CAD build for the part. Positions are in the model's coordinates, mm. Round coordinates to 2 decimals unless told otherwise and drop trailing zeros. Write each loop counter-clockwise with the first axis right and the second up, starting at its lowest first coordinate (ties: lowest second). Pieces come first, ordered by that corner, then holes. Notation, with made-up numbers: (-3, -39) - (25, -39) arc R27 ccw to (25, -2) - close; hole circle Ø7 at (-10, -40). An arc over 180 degrees is marked (long way). Use one line per item in the form item = value. Start each with the question number.
Item 1: Pin check, flat tips, straight feed: pin 1 (5.5 mm diameter, centred on x = -22, z = 217.92, fed in from -Y); pin 2 (2 mm diameter, centred on y = 83, z = 282, fed in from +X); pin 3 (2 mm diameter, centred on x = -8.5, z = 222.5, fed in from -Y). Stop position of each tip, or through.
Item 2: Band-saw the part on B-B, the plane z = 260. List the corners of the cut face in (x, y), and give its area (3 significant figures).
Item 3: Drill centre lines: L1, parallel to X at y = 80.9, z = 303; L2, parallel to Z at x = -35, y = 81.4; L3, parallel to Z at x = 16, y = 80.25. Where is each one in solid material? Low to high.
Item 4: Band-saw the part on D-D, the plane x = 2.5. List the corners of the cut face in (y, z).
Item 5: Band-saw the part on A-A, the plane x = 22. Give the number of separate pieces and of enclosed holes in the cut face, and give its area (3 significant figures).
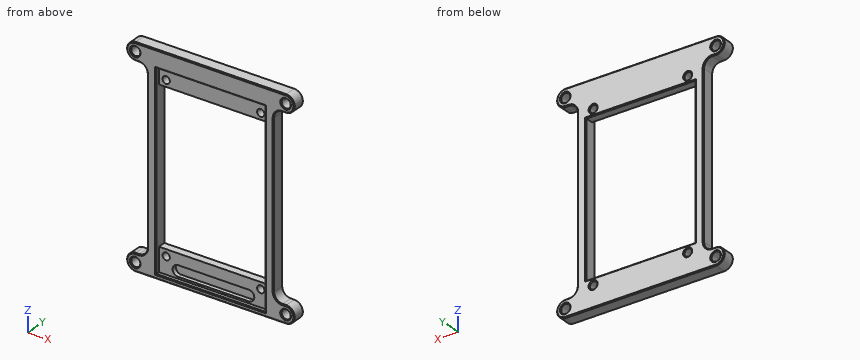
from build123d import *

# Parameters (mm, degrees)
SKETCH210_W     = 58.8
SKETCH210_H     = 99
SKETCH210_R     = 1.7
SKETCH210_W_2   = 50.8
SKETCH210_H_2   = 70
PAD109_DEPTH    = 6
SKETCH211_R     = 2.1
PAD110_DEPTH    = 6
SKETCH212_W     = 50.8
SKETCH212_H     = 89
POCKET044_DEPTH = 2
POCKET045_DEPTH = 2
FILLET_R        = 4
CHAMFER074_SIZE = 0.4


with BuildPart() as part:
    # Sketch210 (on Binder) → Pad109 (new body)
    with BuildSketch(Plane(origin=(0, 78, 0), x_dir=(-1, 0, 0), z_dir=(0, 1, 0))):
        with Locations((0, 257.5)):
            Rectangle(SKETCH210_W, SKETCH210_H)
        with Locations((-22, 217.92)):
            Circle(SKETCH210_R, mode=Mode.SUBTRACT)
        with Locations((22, 217.92)):
            Circle(SKETCH210_R, mode=Mode.SUBTRACT)
        with Locations((22, 294)):
            Circle(SKETCH210_R, mode=Mode.SUBTRACT)
        with Locations((-22, 294)):
            Circle(SKETCH210_R, mode=Mode.SUBTRACT)
        with Locations((0, 256)):
            Rectangle(SKETCH210_W_2, SKETCH210_H_2, mode=Mode.SUBTRACT)
    extrude(amount=PAD109_DEPTH)

    # Sketch211 (on Face13 of Pad109) → Pad110 (join)
    with BuildSketch(Plane.XZ.offset(-78)):
        with BuildLine():
            ThreePointArc((-29.4, 299), (-25.4, 303), (-29.4, 307))
            Line((-29.4, 307), (-35, 307))
            ThreePointArc((-35, 307), (-39, 303), (-35, 299))
            Line((-35, 299), (-29.4, 299))
        make_face()
        with Locations((-35, 303)):
            Circle(SKETCH211_R, mode=Mode.SUBTRACT)
        with BuildLine():
            ThreePointArc((-29.4, 208), (-25.4, 212), (-29.4, 216))
            Line((-29.4, 216), (-35, 216))
            ThreePointArc((-35, 216), (-39, 212), (-35, 208))
            Line((-35, 208), (-29.4, 208))
        make_face()
        with Locations((-35, 212)):
            Circle(SKETCH211_R, mode=Mode.SUBTRACT)
    pad110 = extrude(amount=-PAD110_DEPTH)

    # Mirrored: Pad110 across YZ
    add(pad110.mirror(Plane.YZ))

    # Sketch212 (on Face6 of Mirrored) → Pocket044 (cut)
    with BuildSketch(Plane.XZ.offset(-78)):
        with Locations((0, 254.5)):
            Rectangle(SKETCH212_W, SKETCH212_H)
    extrude(amount=-POCKET044_DEPTH, mode=Mode.SUBTRACT)

    # Sketch213 (on Face28 of Pocket044) → Pocket045 (cut)
    with BuildSketch(Plane.XZ.offset(-80)):
        with BuildLine():
            ThreePointArc((-16.5, 215.9), (-19, 213.4), (-16.5, 210.9))
            Line((-16.5, 210.9), (16.5, 210.9))
            ThreePointArc((16.5, 210.9), (19, 213.4), (16.5, 215.9))
            Line((16.5, 215.9), (-16.5, 215.9))
        make_face()
    extrude(amount=-POCKET045_DEPTH, mode=Mode.SUBTRACT)

    # Fillet
    fillet_edges = [part.edges().sort_by_distance(p)[0] for p in [
        (-29.4, 81, 216),
        (-29.4, 81, 299),
        (29.4, 81, 299),
        (29.4, 81, 216),
    ]]
    fillet(fillet_edges, radius=FILLET_R)

    # Chamfer074
    chamfer074_edges = [part.edges().sort_by_distance(p)[0] for p in [
        (34.2, 84, 216),
        (30.571573, 84, 217.171573),
        (39, 84, 212),
        (29.4, 84, 257.5),
        (0, 84, 208),
        (30.571573, 84, 297.828427),
        (-39, 84, 212),
        (34.2, 84, 299),
        (-34.2, 84, 216),
        (39, 84, 303),
        (-30.571573, 84, 217.171573),
        (0, 84, 307),
        (-29.4, 84, 257.5),
        (-39, 84, 303),
        (-30.571573, 84, 297.828427),
        (-34.2, 84, 299),
        (0, 84, 291),
        (-25.4, 84, 256),
        (0, 84, 221),
        (25.4, 84, 256),
        (-37.1, 84, 212),
        (-37.1, 84, 303),
        (37.1, 84, 212),
        (37.1, 84, 303),
        (-20.3, 84, 294),
        (23.7, 84, 294),
        (-20.3, 84, 217.92),
        (23.7, 84, 217.92),
        (34.2, 78, 216),
        (30.571573, 78, 217.171573),
        (39, 78, 212),
        (29.4, 78, 257.5),
        (0, 78, 208),
        (30.571573, 78, 297.828427),
        (-39, 78, 212),
        (34.2, 78, 299),
        (-34.2, 78, 216),
        (39, 78, 303),
        (-30.571573, 78, 217.171573),
        (0, 78, 307),
        (-29.4, 78, 257.5),
        (-39, 78, 303),
        (-30.571573, 78, 297.828427),
        (-34.2, 78, 299),
        (-37.1, 78, 303),
        (-37.1, 78, 212),
        (37.1, 78, 303),
        (25.4, 78, 254.5),
        (0, 78, 299),
        (-25.4, 78, 254.5),
        (0, 78, 210),
        (37.1, 78, 212),
    ]]
    chamfer(chamfer074_edges, length=CHAMFER074_SIZE)


solid = part.part
Determined:
q1.pin_1 = 80
q1.pin_2 = 29.4
q1.pin_3 = through
q2.outline = (-29.4, 78.4) - (-29, 78) - (-25.8, 78) - (-25.4, 78.4) - (-25.4, 83.6) - (-25.8, 84) - (-29, 84) - (-29.4, 83.6) - close; (25.4, 78.4) - (25.8, 78) - (29, 78) - (29.4, 78.4) - (29.4, 83.6) - (29, 84) - (25.8, 84) - (25.4, 83.6) - close
q2.area = 47.4 mm²
q3.L1 = -39 to -37.1, -32.9 to 32.9, 37.1 to 39
q3.L2 = 208 to 209.9, 214.1 to 216, 299 to 300.9, 305.1 to 307
q3.L3 = 208 to 210.9, 215.9 to 221, 291 to 307
q4.outline = (78, 208.4) - (78.4, 208) - (83.6, 208) - (84, 208.4) - (84, 220.6) - (83.6, 221) - (80, 221) - (80, 215.9) - (82, 215.9) - (82, 210.9) - (80, 210.9) - (80, 210) - (78.4, 210) - (78, 209.6) - close; (78, 299.4) - (78.4, 299) - (80, 299) - (80, 291) - (83.6, 291) - (84, 291.4) - (84, 306.6) - (83.6, 307) - (78.4, 307) - (78, 306.6) - close
q5.separate_pieces = 4
q5.enclosed_holes = 0
q5.area = 108 mm²
